from build123d import *

# Parameters (mm, degrees)
SKETCH_1_R      = 1.65
EXTRUDE_1_DEPTH = 144


with BuildPart() as part:
    # ｽｹｯﾁ1 → ﾎﾞｽ - 押し出し1 (new body)
    with BuildSketch(Plane(origin=(0, 0, 0), x_dir=(0, 0, -1), z_dir=(1, 0, 0))):
        with BuildLine():
            Line((0.5, 0), (2.35, 0))
            ThreePointArc((2.35, 0), (2.703553391, 0.146446609), (2.85, 0.5))
            Line((2.85, 0.5), (2.85, 1))
            ThreePointArc((2.85, 1), (2.703553391, 1.353553391), (2.35, 1.5))
            Line((2.35, 1.5), (1.35, 1.5))
            ThreePointArc((1.35, 1.5), (0.996446609, 1.646446609), (0.85, 2))
            Line((0.85, 2), (0.85, 4.7))
            ThreePointArc((0.85, 4.7), (0.996446609, 5.053553391), (1.35, 5.2))
            Line((1.35, 5.2), (2.35, 5.2))
            ThreePointArc((2.35, 5.2), (2.703553391, 5.346446609), (2.85, 5.7))
            Line((2.85, 5.7), (2.85, 6.5))
            ThreePointArc((2.85, 6.5), (2.996446609, 6.853553391), (3.35, 7))
            Line((3.35, 7), (6.65, 7))
            ThreePointArc((6.65, 7), (7.003553391, 6.853553391), (7.15, 6.5))
            Line((7.15, 6.5), (7.15, 5.7))
            ThreePointArc((7.15, 5.7), (7.296446609, 5.346446609), (7.65, 5.2))
            Line((7.65, 5.2), (8.65, 5.2))
            ThreePointArc((8.65, 5.2), (9.003553391, 5.053553391), (9.15, 4.7))
            Line((9.15, 4.7), (9.15, 2))
            ThreePointArc((9.15, 2), (9.003553391, 1.646446609), (8.65, 1.5))
            Line((8.65, 1.5), (7.65, 1.5))
            ThreePointArc((7.65, 1.5), (7.296446609, 1.353553391), (7.15, 1))
            Line((7.15, 1), (7.15, 0.5))
            ThreePointArc((7.15, 0.5), (7.296446609, 0.146446609), (7.65, 0))
            Line((7.65, 0), (9.5, 0))
            ThreePointArc((9.5, 0), (9.853553391, 0.146446609), (10, 0.5))
            Line((10, 0.5), (10, 19.5))
            ThreePointArc((10, 19.5), (9.853553391, 19.853553391), (9.5, 20))
            Line((9.5, 20), (7.65, 20))
            ThreePointArc((7.65, 20), (7.296446609, 19.853553391), (7.15, 19.5))
            Line((7.15, 19.5), (7.15, 19))
            ThreePointArc((7.15, 19), (7.296446609, 18.646446609), (7.65, 18.5))
            Line((7.65, 18.5), (8.65, 18.5))
            ThreePointArc((8.65, 18.5), (9.003553391, 18.353553391), (9.15, 18))
            Line((9.15, 18), (9.15, 15.3))
            ThreePointArc((9.15, 15.3), (9.003553391, 14.946446609), (8.65, 14.8))
            Line((8.65, 14.8), (7.65, 14.8))
            ThreePointArc((7.65, 14.8), (7.296446609, 14.653553391), (7.15, 14.3))
            Line((7.15, 14.3), (7.15, 13.5))
            ThreePointArc((7.15, 13.5), (7.003553391, 13.146446609), (6.65, 13))
            Line((6.65, 13), (3.35, 13))
            ThreePointArc((3.35, 13), (2.996446609, 13.146446609), (2.85, 13.5))
            Line((2.85, 13.5), (2.85, 14.3))
            ThreePointArc((2.85, 14.3), (2.703553391, 14.653553391), (2.35, 14.8))
            Line((2.35, 14.8), (1.35, 14.8))
            ThreePointArc((1.35, 14.8), (0.996446609, 14.946446609), (0.85, 15.3))
            Line((0.85, 15.3), (0.85, 18))
            ThreePointArc((0.85, 18), (0.996446609, 18.353553391), (1.35, 18.5))
            Line((1.35, 18.5), (2.35, 18.5))
            ThreePointArc((2.35, 18.5), (2.703553391, 18.646446609), (2.85, 19))
            Line((2.85, 19), (2.85, 19.5))
            ThreePointArc((2.85, 19.5), (2.703553391, 19.853553391), (2.35, 20))
            Line((2.35, 20), (0.5, 20))
            ThreePointArc((0.5, 20), (0.146446609, 19.853553391), (0, 19.5))
            Line((0, 19.5), (0, 0.5))
            ThreePointArc((0, 0.5), (0.146446609, 0.146446609), (0.5, 0))
        make_face()
        with Locations((5, 10)):
            Circle(SKETCH_1_R, mode=Mode.SUBTRACT)
    extrude(amount=EXTRUDE_1_DEPTH)


solid = part.part
Design review of the part built by this model. Coordinates are the model's own, in mm. A direction names the side the tool comes from. Round coordinates to 2 decimals unless told otherwise and drop trailing zeros. Loops run counter-clockwise (first coordinate to the right, second up) from the corner with the lowest first, then second, coordinate; pieces in that order, holes last. Notation, with made-up numbers: (47.25, -10.5) - (51.25, -10.5) arc R19 cw to (51.25, -2.5) - close; hole circle Ø4 at (24.25, 22.5). An arc over 180 degrees is marked (long way). One line per question, with ' | ' between items.
1. For faces 4 (the face through (71, 7, -5)), 5 (the face through (71, 17, -9.15)), 6 (the face through (71, 10, -10)), list the 3-axis set-ups (+Z, -Z, +X, -X, +Y, -Y) from which the entire face can be reached by the end or side of a thin tool; tool diameter is ignored.
Results are:
face 4: +X, -X, -Y | face 5: +X, -X | face 6: -Z, +X, -X, +Y, -Y
2. Draft analysis for pull direction Y (two halves, no side actions). For faces 1 (the face through (71, 13, -5)), 2 (the face through (0, 10, -3)), 3 (the face through (71, 17, -0.85)), state which applies: released by +Y, released by -Y, zero draft, split by the parting line, or undercut.
Results are:
face 1: released by +Y | face 2: zero draft | face 3: undercut
3. We need section A-A, the plane y = 16.5. State the section outline as (x, z) points.
Results are:
outline: (0, -10) - (144, -10) - (144, -9.15) - (0, -9.15) - close; (0, -0.85) - (144, -0.85) - (144, 0) - (0, 0) - close
4. For L1, parallel to Y at x = 33.5, z = -2; L2, parallel to Z at x = 29, y = 1; L3, parallel to Z at x = 37.5, y = 3.75, list the stretches that pass through material, from the lowest coordinate up. Write a range as [from, to].
Results are:
L1: y = [0, 1.5], [5.2, 14.8], [18.5, 20] | L2: z = [-10, -7.15], [-2.85, 0] | L3: z = [-10, -9.15], [-0.85, 0]
5. Clearance check with flat-ended pins moving along their axes: P1, Ø3, axis at x = 19.5, z = -1.5, coming from the -Y side; P2, Ø1.5, axis at x = 121.5, z = -6, coming from the +Y side. State where each tip first meets the part, or that it passes through.
Results are:
P1: stops at y = 0 | P2: stops at y = 13.01
6. We need section B-B, the plane z = -5. State the section outline as (x, y) points.
Results are:
outline: (0, 7) - (144, 7) - (144, 8.35) - (0, 8.35) - close; (0, 11.65) - (144, 11.65) - (144, 13) - (0, 13) - close
